from build123d import *

# Parameters (mm, degrees)
ESQUISSE1_W                                    = 65
ESQUISSE1_H                                    = 55
BOSS_EXTRU_1_DEPTH                             = 5
ESQUISSE2_R                                    = 2
ENL_V_MAT_EXTRU_1_DEPTH                        = 86.293610546
FRAISAGE_POUR_VIS_T_TE_FRAIS_E_M41_D           = 4.5
FRAISAGE_POUR_VIS_T_TE_FRAIS_E_M41_CSINK_D     = 9.4
FRAISAGE_POUR_VIS_T_TE_FRAIS_E_M41_CSINK_ANGLE = 90
ESQUISSE6_W                                    = 10.600064569
ESQUISSE6_H                                    = 4.5
ENL_V_MAT_EXTRU_2_DEPTH                        = 86.293610546


with BuildPart() as part:
    # Esquisse1 → Boss.-Extru.1 (new body)
    with BuildSketch(Plane.XY):
        with Locations((32.5, 27.5)):
            Rectangle(ESQUISSE1_W, ESQUISSE1_H)
    extrude(amount=BOSS_EXTRU_1_DEPTH)

    # Esquisse2 → Enl_v. mat.-Extru.1 (cut, through all)
    with BuildSketch(Plane.XY.offset(5)):
        with Locations((5, 27.5)):
            Circle(ESQUISSE2_R)
        with Locations(Location((60, 27.5, 0), (0, 0, 180))):
            Circle(ESQUISSE2_R)
    extrude(amount=-ENL_V_MAT_EXTRU_1_DEPTH, mode=Mode.SUBTRACT)

    # Fraisage pour vis _ t_te frais_e M41 (through all)
    with Locations(Plane.XY.offset(5)):
        with Locations((5, 27.5), (60, 27.5)):
            CounterSinkHole(FRAISAGE_POUR_VIS_T_TE_FRAIS_E_M41_D / 2, FRAISAGE_POUR_VIS_T_TE_FRAIS_E_M41_CSINK_D / 2, counter_sink_angle=FRAISAGE_POUR_VIS_T_TE_FRAIS_E_M41_CSINK_ANGLE)

    # Esquisse6 → Enl_v. mat.-Extru.2 (cut, through all)
    with BuildSketch(Plane.XY.offset(5)):
        with Locations((28.468386436, 11.25)):
            Rectangle(ESQUISSE6_W, ESQUISSE6_H)
    extrude(amount=-ENL_V_MAT_EXTRU_2_DEPTH, mode=Mode.SUBTRACT)


solid = part.part
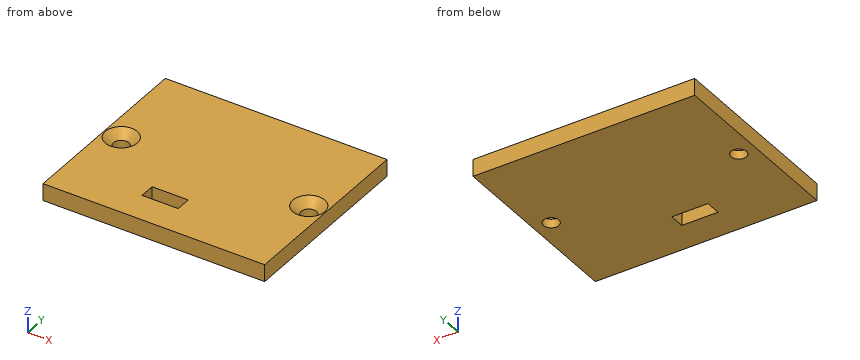
Could you check a few things on this model? Use its own coordinates, in mm. Coordinates: 2 decimals unless noted, no trailing zeros. Loops run counter-clockwise (first coordinate to the right, second up) from the corner with the lowest first, then second, coordinate; pieces in that order, holes last.
1. Imagine slicing it at C-C (x = 5). Please give me the cut outline in (y, z), and give its area (3 significant figures).
2. Imagine slicing it at A-A (y = 27.5). Please give me the cut outline in (x, z).
3. I need wall thicknesses on L1, parallel to X at y = 27.5, z = 2; L2, parallel to Y at x = 60, z = 1.5; L3, parallel to Y at x = 32, z = 2.3. Which ranges of each line are inside material? Lowest first, please.
4. Imagine slicing it at B-B (z = 1.1). Please give me the cut outline in (x, y), and give its area (3 significant figures).
5. Imagine slicing it at D-D (z = 4.3). Please give me the cut outline in (x, y).
6. For P1, Ø1.5, axis at x = 28, z = 4, coming from the -Y side, with a flat end and sliding along its axis, tell me the tip position at first contact or that it passes through.
Computed values:
1. outline: (0, 0) - (25.25, 0) - (25.25, 2.55) - (22.8, 5) - (0, 5) - close; (29.75, 0) - (55, 0) - (55, 5) - (32.2, 5) - (29.75, 2.55) - close
1. area: 246 mm2
2. outline: (0, 0) - (2.75, 0) - (2.75, 2.55) - (0.3, 5) - (0, 5) - close; (7.25, 0) - (57.75, 0) - (57.75, 2.55) - (55.3, 5) - (9.7, 5) - (7.25, 2.55) - close; (62.25, 0) - (65, 0) - (65, 5) - (64.7, 5) - (62.25, 2.55) - close
3. L1: x = 0 to 2.75, 7.25 to 57.75, 62.25 to 65
3. L2: y = 0 to 25.25, 29.75 to 55
3. L3: y = 0 to 9, 13.5 to 55
4. outline: (0, 0) - (65, 0) - (65, 55) - (0, 55) - close; hole circle Ø4.5 at (5, 27.5); hole (23.17, 9) - (33.77, 9) - (33.77, 13.5) - (23.17, 13.5) - close; hole circle Ø4.5 at (60, 27.5)
4. area: 3,500 mm2
5. outline: (0, 0) - (65, 0) - (65, 55) - (0, 55) - close; hole circle Ø8 at (5, 27.5); hole (23.17, 9) - (33.77, 9) - (33.77, 13.5) - (23.17, 13.5) - close; hole circle Ø8 at (60, 27.5)
6. P1: stops at y = 0
